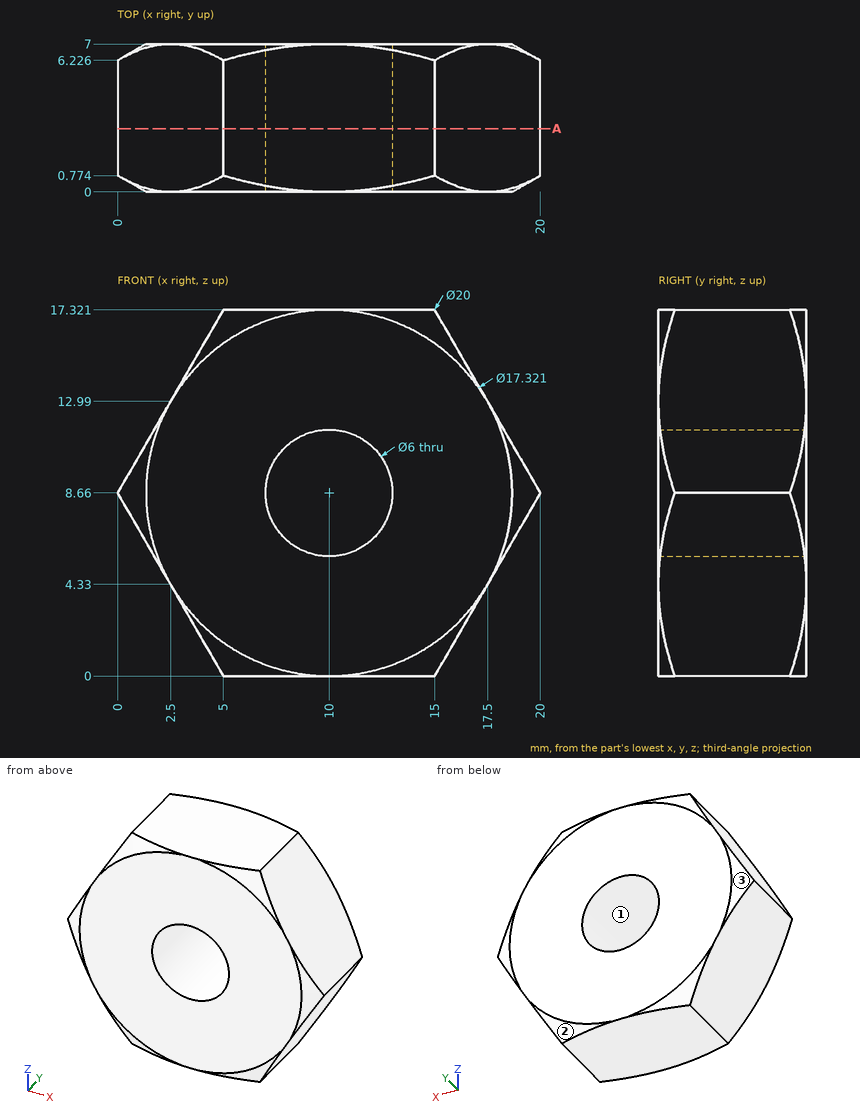
Geometry check sheet. Reference: drawing and pictorial views, mm from the part's lowest x, y, z. Round coordinates to 2 decimals unless told otherwise and drop trailing zeros. Loops run counter-clockwise (first coordinate to the right, second up) from the corner with the lowest first, then second, coordinate; pieces in that order, holes last. Notation, with made-up numbers: (-27, -33.75) - (24, -33.75) arc R33 cw to (24, 0.25) - close; hole circle Ø3 at (29.5, -19). An arc over 180 degrees is marked (long way). Answer in a Markdown table with one row per item. Add a question column.
Q1. Gauge pin test, flat ends, axial feed: pin 1 (2 mm diameter, centred on y = 6, z = 12.5, fed in from +X); pin 2 (4 mm diameter, centred on x = 3.5, y = 6, fed in from +Z); pin 3 (3 mm diameter, centred on y = 1, z = 5.5, fed in from -X); pin 4 (3.5 mm diameter, centred on x = 10, z = 8.66, fed in from +Y). Record the tip position at first contact, or that the pin passes through.
Q2. Material ranges on line 1 (X direction, y = 2.5, z = 9.75) (1 decimal); line 2 (Z direction, x = 18, y = 3.25) (1 decimal); line 3 (X direction, y = 4.5, z = 13.75), recorded low to high.
Q3. Section check A-A on y = 3. Enter the section's corners in (x, z).
Q4. Release check for a two-part mould opening along Z. For the marked faces 1, 2 and 3 record: pulls with the +Z half, pulls with the -Z half, needs draft (parallel to the pull), parting line crosses it, or undercut.
Found:
| question | item | result |
|---|---|---|
| 1 | pin 1 | stops at x = 18.36 |
| 1 | pin 2 | stops at z = 17.32 |
| 1 | pin 3 | stops at x = 0.96 |
| 1 | pin 4 | passes through |
| 2 | line 1 | x = 0.6 to 7.2, 12.8 to 19.4 |
| 2 | line 2 | z = 5.2 to 12.1 |
| 2 | line 3 | x = 2.94 to 17.06 |
| 3 | outline | (0, 8.66) - (5, 0) - (15, 0) - (20, 8.66) - (15, 17.32) - (5, 17.32) - close; hole circle Ø6 at (10, 8.66) |
| 4 | face 1 | undercut |
| 4 | face 2 | pulls with the -Z half |
| 4 | face 3 | parting line crosses it |
